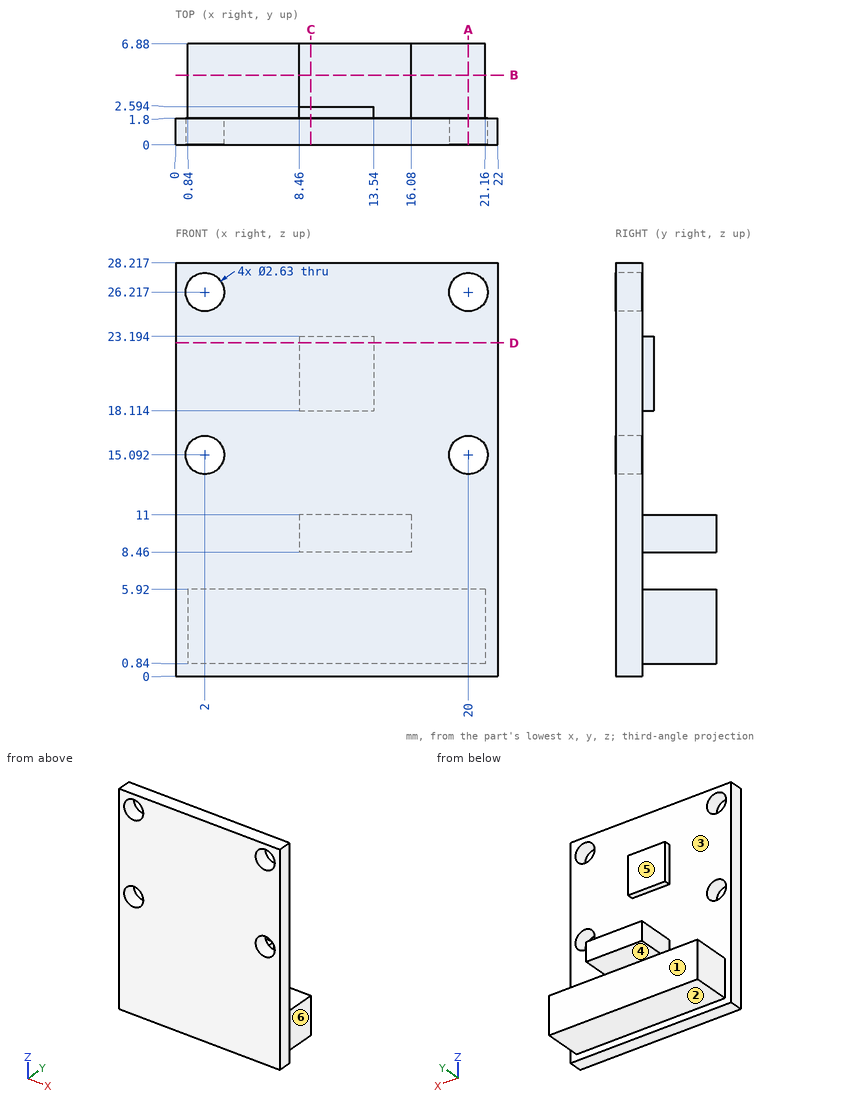
For this review, use the dimensioned drawing (mm, ordinates from the lowest corner) and the shaded views. A direction names the side the tool comes from. Coordinates: 2 decimals unless noted, no trailing zeros. Loops run counter-clockwise (first coordinate to the right, second up) from the corner with the lowest first, then second, coordinate; pieces in that order, holes last.
1. Add section B-B, the plane y = 4.75. Give the boundary of the cut face in (x, z), then the cut area to 3 significant figures.
2. Mouldability with a two-part tool opening along Z and no side actions: class the marked faces 1, 2 and 3 as +Z half, -Z half, draft (parallel to the pull), parting line (faces both ways), or undercut.
3. Add section C-C, the plane x = 9.25. Give the boundary of the cut face in (y, z).
4. Add section A-A, the plane x = 20. Give the boundary of the cut face in (y, z).
5. Add section D-D, the plane z = 22.75. Give the boundary of the cut face in (x, y).
6. For the marked faces 4, 5 and 6, list the 3-axis set-ups (+Z, -Z, +X, -X, +Y, -Y) from which the entire face can be reached by the end or side of a thin tool; tool diameter is ignored.
7. Insertion check: P1, Ø1.6, axis at x = 2, z = 26.22, coming from the -Y side; P2, Ø1.5, axis at x = 11.5, y = 3.5, coming from the +Z side; P3, Ø1.5, axis at y = 5, z = 2.5, coming from the -X side; P4, Ø4, axis at x = 7.5, y = 4.5, coming from the -Z side. Each pin has a flat end and moves straight along its axis. Give the tip position at first contact, or say it passes through.
8. For line 1 (Z direction, x = 2, y = 1.35); line 2 (X direction, y = 1.5, z = 26); line 3 (Z direction, x = 9.25, y = 4), list the stretches that pass through material, from the lowest coordinate up.
Result:
1. outline: (0.84, 0.84) - (21.16, 0.84) - (21.16, 5.92) - (0.84, 5.92) - close; (8.46, 8.46) - (16.08, 8.46) - (16.08, 11) - (8.46, 11) - close
1. area: 123 mm2
2. face 1: draft
2. face 2: -Z half
2. face 3: undercut
3. outline: (0, 0) - (1.8, 0) - (1.8, 0.84) - (6.88, 0.84) - (6.88, 5.92) - (1.8, 5.92) - (1.8, 8.46) - (6.88, 8.46) - (6.88, 11) - (1.8, 11) - (1.8, 18.11) - (2.59, 18.11) - (2.59, 23.19) - (1.8, 23.19) - (1.8, 28.22) - (0, 28.22) - close
4. outline: (0, 0) - (1.8, 0) - (1.8, 0.84) - (6.88, 0.84) - (6.88, 5.92) - (1.8, 5.92) - (1.8, 13.78) - (0, 13.78) - close; (0, 16.41) - (1.8, 16.41) - (1.8, 24.9) - (0, 24.9) - close; (0, 27.53) - (1.8, 27.53) - (1.8, 28.22) - (0, 28.22) - close
5. outline: (0, 0) - (22, 0) - (22, 1.8) - (13.54, 1.8) - (13.54, 2.59) - (8.46, 2.59) - (8.46, 1.8) - (0, 1.8) - close
6. face 4: +X, -X, +Y
6. face 5: +Z, +X, -X, +Y
6. face 6: +Z, -Z, +X, +Y
7. P1: passes through
7. P2: stops at z = 11
7. P3: stops at x = 0.84
7. P4: stops at z = 0.84
8. line 1: z = 0 to 13.78, 16.41 to 24.9, 27.53 to 28.22
8. line 2: x = 0 to 0.7, 3.3 to 18.7, 21.3 to 22
8. line 3: z = 0.84 to 5.92, 8.46 to 11
